Input: part model. Units: mm. Frame: model coordinates. A direction names the side the tool comes from. Give positions to 0.01 mm unless a question says otherwise; leave off trailing zeros. Use a Markdown table: item, result.
from build123d import *
from OCP.BRepAlgoAPI import BRepAlgoAPI_Cut
from OCP.TopTools import TopTools_ListOfShape

# Parameters (mm, degrees)
SKETCH1_RX              = 238.176778745998
SKETCH1_RY              = 100
SKETCH1_R               = 9.000000000000009
SKETCH1_W               = 152.4
SKETCH1_H               = 77
BOSS_EXTRUDE1_DEPTH     = 719.5500000000001
CUT_EXTRUDE1_DEPTH      = 771.8388550363948
CUT_EXTRUDE1_DEPTH_BACK = 771.8388550363948
FILLET1_R               = 9.999999999999996
BOSS_EXTRUDE2_REACH     = 780.772
SKETCH4_W               = 152.4
SKETCH4_H               = 277.7592603894774
CUT_EXTRUDE2_DEPTH      = 771.8388551788538
CUT_EXTRUDE2_DEPTH_BACK = 771.8388551788538
SKETCH5_R               = 2.7500000000000084
SKETCH5_R_2             = 8.50000000000001


with BuildPart() as part:
    # Sketch1 → Boss-Extrude1 (new body)
    with BuildSketch(Plane.XY):
        with Locations(Location((0, 40.399999999999984), (0, 0, 6.84e-15))):
            Ellipse(SKETCH1_RX, SKETCH1_RY)
        with Locations((173.785, 25.400000000000006)):
            Circle(SKETCH1_R, mode=Mode.SUBTRACT)
        with Locations(Location((-173.785, 25.400000000000006, 0), (0, 0, 180))):
            Circle(SKETCH1_R, mode=Mode.SUBTRACT)
        Polygon((-123.39999999999999, 119.29999999999997), (123.39999999999999, 119.3), (123.4, 68.5), (-123.4, 68.49999999999997), align=None, mode=Mode.SUBTRACT)
        Rectangle(SKETCH1_W, SKETCH1_H, mode=Mode.SUBTRACT)
    extrude(amount=BOSS_EXTRUDE1_DEPTH)

    # Sketch3 → Cut-Extrude1 (cut, two sides: drawn at the far end of the back side and taken through both)
    with BuildSketch(Plane(origin=(0, 0, 0), x_dir=(0, 0, -1), z_dir=(1, 0, 0)).offset(-CUT_EXTRUDE1_DEPTH_BACK)):
        Polygon((1280.4819340937215, -287.25956976454023), (-201.17484480506153, -72.00000000000001), (-731.1748448050615, 4.999999999999994), (-2212.831623703845, 220.2595697645402), (-2643.350763232925, -2743.053988033026), (849.9627945646412, -3250.5731275621065), align=None)
    extrude(amount=CUT_EXTRUDE1_DEPTH + CUT_EXTRUDE1_DEPTH_BACK, mode=Mode.SUBTRACT)

    # Fillet1
    fillet1_edges = [part.edges().sort_by_distance(p)[0] for p in [
        (148.69467604524613, 3.311107452849548, 719.5500000000004),
        (-148.69467604524613, 3.311107452849548, 719.5500000000004),
    ]]
    fillet(fillet1_edges, radius=FILLET1_R)

    # Sketch4 → Boss-Extrude2 (add, up to next)
    with BuildSketch(Plane(origin=(0, -38.5, 0), x_dir=(1, 0, 0), z_dir=(0, 1, 0)), mode=Mode.PRIVATE) as boss_extrude2_sk1:
        with Locations((0, -292.8796301947387)):
            Rectangle(SKETCH4_W, SKETCH4_H)
    boss_extrude2_tool1 = extrude(boss_extrude2_sk1.sketch, amount=BOSS_EXTRUDE2_REACH, mode=Mode.PRIVATE) - part.part
    add(boss_extrude2_tool1.solids().sort_by_distance((0, -38.5, 292.87963))[0])


with BuildPart() as cut_extrude2_tool:
    # Sketch5 → Cut-Extrude2 (new, two sides: drawn at the far end of the back side and taken through both)
    with BuildSketch(Plane(origin=(0, 0, 0), x_dir=(0, 0, -1), z_dir=(1, 0, 0)).offset(-CUT_EXTRUDE2_DEPTH_BACK)):
        with Locations((-179.00000000000003, 53.5)):
            Circle(SKETCH5_R)
        with Locations((-89.00000000000003, 53.5)):
            Circle(SKETCH5_R_2)
    extrude(amount=CUT_EXTRUDE2_DEPTH + CUT_EXTRUDE2_DEPTH_BACK)


with BuildPart() as part_1:
    add(part.part)

    # Cut-Extrude2: cut by cut_extrude2_tool, with a tolerance
    cut_extrude2_stock = TopTools_ListOfShape()
    cut_extrude2_stock.Append(part_1.part.wrapped)
    cut_extrude2_tools = TopTools_ListOfShape()
    cut_extrude2_tools.Append(cut_extrude2_tool.part.wrapped)
    cut_extrude2_cut = BRepAlgoAPI_Cut()
    cut_extrude2_cut.SetArguments(cut_extrude2_stock)
    cut_extrude2_cut.SetTools(cut_extrude2_tools)
    cut_extrude2_cut.SetFuzzyValue(0.00001)
    cut_extrude2_cut.Build()
    add(Compound.cast(cut_extrude2_cut.Shape()).solids(), mode=Mode.REPLACE)


solid = part_1.part
1) First-contact query: pin 1 Ø10 at (y, z) = (53.5, 89) entering from +X; pin 2 Ø12 at (x, z) = (-28, 592.5) entering from -Y; pin 3 Ø3 at (x, z) = (-59.5, 99) entering from -Y; pin 4 Ø1 at (x, z) = (-82, 426.5) entering from -Y. Flat tips, straight axial feed; report the tip coordinate or a pass-through.
Response values:
| item | result |
|---|---|
| pin 1 | passes through |
| pin 2 | stops at y = 38.5 |
| pin 3 | stops at y = -56.59 |
| pin 4 | stops at y = -39.34 |
2) Cut plane A-A on z = 124. State how many separate pieces and enclosed holes the cut face has, and give its area (3 significant figures).
Response values:
| item | result |
|---|---|
| separate pieces | 1 |
| enclosed holes | 4 |
| area | 50,000 mm² |
3) Mould query, pull axis X, two halves, no side actions, for faces 6 (the face through (-123.4, 94, 355)), 7 (the face through (-3, 63, 719.55)). Classes: released by +X, released by -X, zero draft, split by the parting line, or undercut.
Response values:
| item | result |
|---|---|
| face 6 | undercut |
| face 7 | zero draft |
4) Reachability of faces 1 (the face through (-1, -38.5, 76)), 2 (the face through (2, 68.5, 355)), 3 (the face through (94.69, -29.198, 495.785)), 4 (the face through (-76.2, 8, 542)), 5 (the face through (-3.33, 53.87, 97.49)) from +Z, -Z, +X, -X, +Y, -Y: full face, straight path, thin tool, end or side. Return the list, or none.
Response values:
| item | result |
|---|---|
| face 1 | -Z |
| face 2 | +Z, -Z |
| face 3 | +Z, +X, -X, -Y |
| face 4 | +Z, -Y |
| face 5 | +X, -X |
5) Material intervals for line 1 (Z direction, x = -95.5, y = 53.5); line 2 (Y direction, x = 44, z = 179); line 3 (Y direction, x = 101, z = 89), sorted ascending. Write a range as from..to.
Response values:
| item | result |
|---|---|
| line 1 | z = 0..80.5, 97.5..176.25, 181.75..719.55 |
| line 2 | y = -57.88..50.75, 56.25..68.5, 119.3..138.68 |
| line 3 | y = -50.16..45, 62..68.5, 119.3..130.96 |
